Source: CAD feature listing. Evaluate the final solid. Frame: model axes, mm. A direction names the side the tool comes from. Give positions to 0.01 mm unless a question says otherwise; leave off trailing zeros. Write each loop counter-clockwise with the first axis right and the second up, starting at its lowest first coordinate (ties: lowest second). Pieces come first, ordered by that corner, then holes. Notation, with made-up numbers: (2, -26.75) -> (61, -26.75) arc R23 ccw to (61, 2.25) -> close; hole circle Ø1 at (87, 81.25). An arc over 180 degrees is marked (long way). Write item = value, one per line.
from build123d import *

# Parameters (mm, degrees)
SKETCH1_R   = 12.7
SKETCH1_R_2 = 0.79375
BASE_DEPTH  = 2.7


with BuildPart() as part:
    # Sketch1 → Base (new body)
    with BuildSketch(Plane(origin=(0, 0, 0), x_dir=(0, 0, -1), z_dir=(1, 0, 0))):
        with Locations(Location((0, 0, 0), (0, 0, 180))):
            Circle(SKETCH1_R)
        with Locations(Location((0, 10.16, 0), (0, 0, 180))):
            Circle(SKETCH1_R_2, mode=Mode.SUBTRACT)
        with Locations(Location((3.888063673, 9.38661605, 0), (0, 0, 180))):
            Circle(SKETCH1_R_2, mode=Mode.SUBTRACT)
        with Locations(Location((7.184204897, 7.184204897, 0), (0, 0, 180))):
            Circle(SKETCH1_R_2, mode=Mode.SUBTRACT)
        with Locations(Location((9.38661605, 3.888063673, 0), (0, 0, 180))):
            Circle(SKETCH1_R_2, mode=Mode.SUBTRACT)
        with Locations(Location((10.16, 0, 0), (0, 0, 180))):
            Circle(SKETCH1_R_2, mode=Mode.SUBTRACT)
        with Locations(Location((9.38661605, -3.888063673, 0), (0, 0, 180))):
            Circle(SKETCH1_R_2, mode=Mode.SUBTRACT)
        with Locations(Location((7.184204897, -7.184204897, 0), (0, 0, 180))):
            Circle(SKETCH1_R_2, mode=Mode.SUBTRACT)
        with Locations(Location((3.888063673, -9.38661605, 0), (0, 0, 180))):
            Circle(SKETCH1_R_2, mode=Mode.SUBTRACT)
        with Locations(Location((0, -10.16, 0), (0, 0, 180))):
            Circle(SKETCH1_R_2, mode=Mode.SUBTRACT)
        with Locations(Location((-3.888063673, -9.38661605, 0), (0, 0, 180))):
            Circle(SKETCH1_R_2, mode=Mode.SUBTRACT)
        with Locations(Location((-7.184204897, -7.184204897, 0), (0, 0, 180))):
            Circle(SKETCH1_R_2, mode=Mode.SUBTRACT)
        with Locations(Location((-9.38661605, -3.888063673, 0), (0, 0, 180))):
            Circle(SKETCH1_R_2, mode=Mode.SUBTRACT)
        with Locations(Location((-10.16, 0, 0), (0, 0, 180))):
            Circle(SKETCH1_R_2, mode=Mode.SUBTRACT)
        with Locations(Location((-9.38661605, 3.888063673, 0), (0, 0, 180))):
            Circle(SKETCH1_R_2, mode=Mode.SUBTRACT)
        with Locations(Location((-7.184204897, 7.184204897, 0), (0, 0, 180))):
            Circle(SKETCH1_R_2, mode=Mode.SUBTRACT)
        with Locations(Location((-3.888063673, 9.38661605, 0), (0, 0, 180))):
            Circle(SKETCH1_R_2, mode=Mode.SUBTRACT)
        with BuildLine():
            Line((1, 0.979795897), (1, -0.979795897))
            ThreePointArc((1, -0.979795897), (0, -1.4), (-1, -0.979795897))
            Line((-1, -0.979795897), (-1, 0.979795897))
            ThreePointArc((-1, 0.979795897), (0, 1.4), (1, 0.979795897))
        make_face(mode=Mode.SUBTRACT)
    extrude(amount=BASE_DEPTH)


solid = part.part
(1) Pull-direction query (Y, two-part tool) for faces 3 (the face through (0, 0, 3)), 4 (the face through (1.331, 3.219, 9.813)); classes: pulls with the +Y half, pulls with the -Y half, needs draft (parallel to the pull), parting line crosses it, or undercut.
Values follow:
face_3 = needs draft
face_4 = undercut
(2) Section query A-A (z = 0). Return loops of the section in (x, y), plus the area to 3 significant figures.
Values follow:
outline = (0, -12.7) -> (2.7, -12.7) -> (2.7, -10.95) -> (0, -10.95) -> close; (0, -9.37) -> (2.7, -9.37) -> (2.7, -1.4) -> (0, -1.4) -> close; (0, 1.4) -> (2.7, 1.4) -> (2.7, 9.37) -> (0, 9.37) -> close; (0, 10.95) -> (2.7, 10.95) -> (2.7, 12.7) -> (0, 12.7) -> close
area = 52.4 mm2
(3) Section query C-C (z = 7.25). Return loops of the section in (x, y).
Values follow:
outline = (0, -10.43) -> (2.7, -10.43) -> (2.7, -7.98) -> (0, -7.98) -> close; (0, -6.39) -> (2.7, -6.39) -> (2.7, 6.39) -> (0, 6.39) -> close; (0, 7.98) -> (2.7, 7.98) -> (2.7, 10.43) -> (0, 10.43) -> close
(4) First-contact query: pin 1 (2 mm diameter, centred on y = 0, z = 10.16, fed in from -X). Flat tip, straight axial feed; report the tip coordinate or a pass-through.
Values follow:
pin_1 = 0
(5) Material intervals for line 1 (Y direction, x = 1.55, z = -10); line 2 (Y direction, x = 0.25, z = 9); line 3 (Y direction, x = 1.95, z = -3.5), sorted ascending.
Values follow:
line_1 = -7.83 to -4.39, -3.38 to -0.78, 0.78 to 3.38, 4.39 to 7.83
line_2 = -8.96 to -4.58, -3.19 to 3.19, 4.58 to 8.96
line_3 = -12.21 to -10.08, -8.69 to 8.69, 10.08 to 12.21
(6) Section query B-B (y = -4.25). Return loops of the section in (x, z), plus the area to 3 significant figures.
Values follow:
outline = (0, -11.97) -> (2.7, -11.97) -> (2.7, -10.09) -> (0, -10.09) -> close; (0, -8.68) -> (2.7, -8.68) -> (2.7, 8.68) -> (0, 8.68) -> close; (0, 10.09) -> (2.7, 10.09) -> (2.7, 11.97) -> (0, 11.97) -> close
area = 57.0 mm2
(7) Section query D-D (x = 1.75). Give the number of separate pieces and of enclosed holes in the cut face, plus the area to 3 significant figures.
Values follow:
separate_pieces = 1
enclosed_holes = 17
area = 470 mm2
(8) Access query for faces 1 (the face through (1.3, 1.4, 0)), 2 (the face through (2.7, 0, 3)). Directions: +Z, -Z, +X, -X, +Y, -Y. A direction counts if a zero-diameter tool reaches every point of the face in a straight line with its end or side. Return the directions, or none.
Values follow:
face_1 = +X, -X
face_2 = +Z, -Z, +X, +Y, -Y
